from build123d import *

# Parameters (mm, degrees)
F0_W     = 1500
F0_H     = 1200
F1_DEPTH = 3
F2_SIZE  = 300
F3_SIZE  = 100
F4_R     = 300
F5_R     = 100


with BuildPart() as f1:
    # F0 (on Top) → F1 (new body)
    with BuildSketch(Plane.XY):
        Rectangle(F0_W, F0_H)
    extrude(amount=F1_DEPTH)

    # F2
    f2_edges = [f1.edges().sort_by_distance(p)[0] for p in [
        (750, -600, 1.5),
        (750, 600, 1.5),
    ]]
    chamfer(f2_edges, length=F2_SIZE)

    # F3
    f3_edges = [f1.edges().sort_by_distance(p)[0] for p in [
        (-750, -600, 1.5),
        (-750, 600, 1.5),
    ]]
    chamfer(f3_edges, length=F3_SIZE)

    # F4
    f4_edges = [f1.edges().sort_by_distance(p)[0] for p in [
        (750, -300, 1.5),
        (450, -600, 1.5),
        (750, 300, 1.5),
        (450, 600, 1.5),
    ]]
    fillet(f4_edges, radius=F4_R)

    # F5
    f5_edges = [f1.edges().sort_by_distance(p)[0] for p in [
        (-750, -500, 1.5),
        (-650, -600, 1.5),
        (-650, 600, 1.5),
        (-750, 500, 1.5),
    ]]
    fillet(f5_edges, radius=F5_R)


solid = f1.part
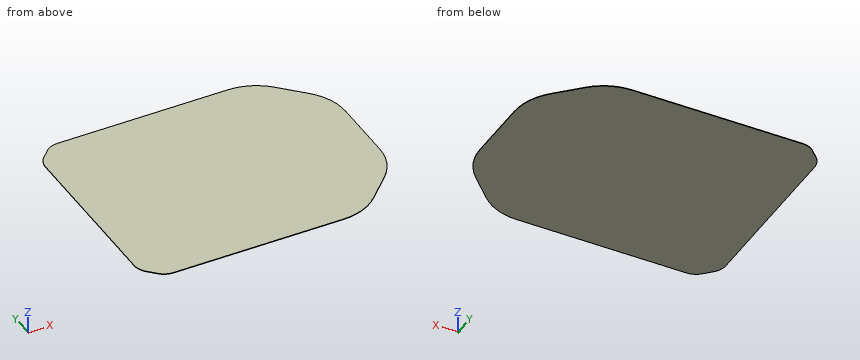
For this review, take the finished solid that the model builds, in its own axes (mm). Give positions to 0.01 mm unless a question says otherwise; leave off trailing zeros. Loops run counter-clockwise (first coordinate to the right, second up) from the corner with the lowest first, then second, coordinate; pieces in that order, holes last.
Item 1: For line 1 along X through (y, z) = (185, 2.3); line 2 along X through (y, z) = (-178.5, 1.45); line 3 along Y through (x, z) = (-628, 2.25), list the stretches that pass through material, from the lowest coordinate up.
Item 2: Insertion check: pin 1 (4 mm diameter, centred on x = 381.5, y = -471.5, fed in from -Z). The pin has a flat end and moves straight along its axis. Give the tip position at first contact, or say it passes through.
Item 3: Take a section at B-B, the plane y = -410. State the section outline as (x, z) points, and give its area (3 significant figures).
Item 4: Take a section at A-A, the plane z = 1.1. State the section outline as (x, y) points.
Item 5: Take a section at C-C, the plane x = 609.5. State the section outline as (y, z) points, and give its area (3 significant figures).
Calculated:
1. line 1: x = -750 to 749.86
1. line 2: x = -750 to 749.99
1. line 3: y = -598.1 to 598.1
2. pin 1: stops at z = 0
3. outline: (-750, 0) - (640, 0) - (640, 3) - (-750, 3) - close
3. area: 4,170 mm2
4. outline: (-750, -458.58) arc R100 ccw to (-720.71, -529.29) - (-679.29, -570.71) arc R100 ccw to (-608.58, -600) - (325.74, -600) arc R300 ccw to (537.87, -512.13) - (662.13, -387.87) arc R300 ccw to (750, -175.74) - (750, 175.74) arc R300 ccw to (662.13, 387.87) - (537.87, 512.13) arc R300 ccw to (325.74, 600) - (-608.58, 600) arc R100 ccw to (-679.29, 570.71) - (-720.71, 529.29) arc R100 ccw to (-750, 458.58) - close
5. outline: (-440.5, 0) - (440.5, 0) - (440.5, 3) - (-440.5, 3) - close
5. area: 2,640 mm2
